Could you check a few things on this model? Use its own coordinates, in mm. Face numbers are marked on the shaded views. A direction names the side the tool comes from. Coordinates: 2 decimals unless noted, no trailing zeros. Write each loop counter-clockwise with the first axis right and the second up, starting at its lowest first coordinate (ties: lowest second). Pieces come first, ordered by that corner, then holes.
Item 1: I want a section at C-C on x = 10.9. Please give me the cut outline in (y, z).
Item 2: Which directions (+Z, -Z, +X, -X, +Y, -Y) give clear straight access to the entire face, cutting with the end or side of a thin tool? Please do the marked faces 5, 6 and 7.
Item 3: For P1, Ø3, axis at y = -27, z = 10.5, coming from the +X side; P2, Ø1.2, axis at y = -17, z = 11.5, coming from the +X side; P3, Ø1.2, axis at y = -16.5, z = 10, coming from the -X side, each with a flat end and sliding along its axis, tell me the tip position at first contact or that it passes through.
Item 4: I want a section at B-B on y = -21.5. Please give me the cut outline in (x, z), then the cut area to 3 significant figures.
Item 5: I want a section at D-D on x = 3.5. Please give me the cut outline in (y, z).
Item 6: I want a section at A-A on x = 19.5. Please give me the cut outline in (y, z).
Item 7: Thinking about a two-plate mould opening in Z: for the marked faces 1, 2, 3 and 4, which applies, +Z half, -Z half, draft (parallel to the pull), parting line (faces both ways), or undercut?
Item 8: If I drill on probe 1 along X at (y, z) = (-10, 10.9); probe 2 along Y at (x, z) = (7.2, 10.9); probe 3 along X at (y, z) = (-11, 14.5), over which ranges is the centre line in solid material (lowest first)?
from build123d import *

# Parameters (mm, degrees)
CROQUIS1_W              = 21.8
CROQUIS1_H              = 35
SALIENTE_EXTRUIR1_DEPTH = 21.8
CROQUIS6_R              = 2
CORTAR_EXTRUIR2_DEPTH   = 21.8
REDONDEO2_R             = 1
REDONDEO3_R             = 4
CROQUIS7_R              = 3.5
CORTAR_EXTRUIR3_DEPTH   = 3
CORTAR_EXTRUIR4_REACH   = 48.642
CROQUIS11_R             = 3.5
CROQUIS11_W             = 3
CROQUIS11_H             = 8.4
MATRIZL1_COUNT          = 2
MATRIZL1_PITCH          = 18.8
CROQUIS14_W             = 3
CROQUIS14_H             = 8.4
SALIENTE_EXTRUIR2_DEPTH = 20
CROQUIS15_W             = 3
CROQUIS15_H             = 8.4
SALIENTE_EXTRUIR3_DEPTH = 20


with BuildPart() as part:
    # Croquis1 → Saliente-Extruir1 (new body)
    with BuildSketch(Plane(origin=(0, 0, 0), x_dir=(0, 0, -1), z_dir=(1, 0, 0))):
        with Locations((-10.9, -17.5)):
            Rectangle(CROQUIS1_W, CROQUIS1_H)
    extrude(amount=SALIENTE_EXTRUIR1_DEPTH)

    # Croquis6 → Cortar-Extruir2 (cut)
    with BuildSketch(Plane.ZY):
        with Locations((10.9, -28)):
            Circle(CROQUIS6_R)
        with Locations((10.9, -17.5)):
            Circle(CROQUIS6_R)
        with Locations(Location((10.9, -7, 0), (0, 0, 180))):
            Circle(CROQUIS6_R)
    extrude(amount=-CORTAR_EXTRUIR2_DEPTH, mode=Mode.SUBTRACT)

    # Redondeo2
    redondeo2_edges = [part.edges().sort_by_distance(p)[0] for p in [
        (21.8, -35, 10.9),
        (21.8, -17.5, 0),
        (21.8, 0, 10.9),
        (0, -17.5, 0),
        (0, -35, 10.9),
        (0, -17.5, 21.8),
        (0, 0, 10.9),
        (21.8, -17.5, 21.8),
    ]]
    fillet(redondeo2_edges, radius=REDONDEO2_R)

    # Redondeo3
    # the kernel refuses this fillet: 4 mm, written as the material it takes off along each edge
    with BuildSketch(Plane(origin=(0, -4, 4), x_dir=(0, 1, 0), z_dir=(0, 0, 1))) as redondeo3_piece_1:
        with BuildLine():
            CenterArc((3, -1), 1, 0, 90)
            Line((4, -1), (4, 0))
            Line((4, 0), (3, 0))
        make_face()
    revolve(axis=Axis((0, -4, 4), (-1, 0, 0)), revolution_arc=90, mode=Mode.SUBTRACT)
    with BuildSketch(Plane(origin=(0, -31, 4), x_dir=(0, 0, -1), z_dir=(0, 1, 0))) as redondeo3_piece_2:
        with BuildLine():
            CenterArc((3, -1), 1, 0, 90)
            Line((4, -1), (4, 0))
            Line((4, 0), (3, 0))
        make_face()
    revolve(axis=Axis((0, -31, 4), (-1, 0, 0)), revolution_arc=90, mode=Mode.SUBTRACT)
    with BuildSketch(Plane(origin=(0, -4, 17.8), x_dir=(0, 0, 1), z_dir=(0, -1, 0))) as redondeo3_piece_3:
        with BuildLine():
            CenterArc((3, -1), 1, 0, 90)
            Line((4, -1), (4, 0))
            Line((4, 0), (3, 0))
        make_face()
    revolve(axis=Axis((0, -4, 17.8), (-1, 0, 0)), revolution_arc=90, mode=Mode.SUBTRACT)
    with BuildSketch(Plane(origin=(0, -31, 17.8), x_dir=(0, -1, 0), z_dir=(0, 0, -1))) as redondeo3_piece_4:
        with BuildLine():
            CenterArc((3, -1), 1, 0, 90)
            Line((4, -1), (4, 0))
            Line((4, 0), (3, 0))
        make_face()
    revolve(axis=Axis((0, -31, 17.8), (-1, 0, 0)), revolution_arc=90, mode=Mode.SUBTRACT)
    with BuildSketch(Plane(origin=(21.8, -4, 4), x_dir=(0, 0, -1), z_dir=(0, -1, 0))) as redondeo3_piece_5:
        with BuildLine():
            CenterArc((3, -1), 1, 0, 90)
            Line((4, -1), (4, 0))
            Line((4, 0), (3, 0))
        make_face()
    revolve(axis=Axis((21.8, -4, 4), (1, 0, 0)), revolution_arc=90, mode=Mode.SUBTRACT)
    with BuildSketch(Plane(origin=(21.8, -31, 4), x_dir=(0, -1, 0), z_dir=(0, 0, 1))) as redondeo3_piece_6:
        with BuildLine():
            CenterArc((3, -1), 1, 0, 90)
            Line((4, -1), (4, 0))
            Line((4, 0), (3, 0))
        make_face()
    revolve(axis=Axis((21.8, -31, 4), (1, 0, 0)), revolution_arc=90, mode=Mode.SUBTRACT)
    with BuildSketch(Plane(origin=(21.8, -4, 17.8), x_dir=(0, 1, 0), z_dir=(0, 0, -1))) as redondeo3_piece_7:
        with BuildLine():
            CenterArc((3, -1), 1, 0, 90)
            Line((4, -1), (4, 0))
            Line((4, 0), (3, 0))
        make_face()
    revolve(axis=Axis((21.8, -4, 17.8), (1, 0, 0)), revolution_arc=90, mode=Mode.SUBTRACT)
    with BuildSketch(Plane(origin=(21.8, -31, 17.8), x_dir=(0, 0, 1), z_dir=(0, 1, 0))) as redondeo3_piece_8:
        with BuildLine():
            CenterArc((3, -1), 1, 0, 90)
            Line((4, -1), (4, 0))
            Line((4, 0), (3, 0))
        make_face()
    revolve(axis=Axis((21.8, -31, 17.8), (1, 0, 0)), revolution_arc=90, mode=Mode.SUBTRACT)
    with BuildSketch(Plane(origin=(0, -35, 21.8), x_dir=(0, 1, 0), z_dir=(1, 0, 0)), Plane(origin=(0, 0, 21.8), x_dir=(0, 0, -1), z_dir=(1, 0, 0))) as redondeo3_piece_9:
        with BuildLine():
            CenterArc((REDONDEO3_R, -REDONDEO3_R), REDONDEO3_R, 90, 90)
            Line((0, -REDONDEO3_R), (0, 0))
            Line((0, 0), (REDONDEO3_R, 0))
        make_face()
    extrude(amount=21.8, mode=Mode.SUBTRACT)
    with BuildSketch(Plane(origin=(0, 0, 0), x_dir=(0, 0, 1), z_dir=(1, 0, 0)), Plane(origin=(0, -35, 0), x_dir=(0, 1, 0), z_dir=(1, 0, 0))) as redondeo3_piece_10:
        with BuildLine():
            CenterArc((REDONDEO3_R, REDONDEO3_R), REDONDEO3_R, 180, 90)
            Line((0, REDONDEO3_R), (0, 0))
            Line((0, 0), (REDONDEO3_R, 0))
        make_face()
    extrude(amount=21.8, mode=Mode.SUBTRACT)

    # Croquis7 → Cortar-Extruir3 (cut)
    with BuildSketch(Plane(origin=(21.8, 0, 0), x_dir=(0, 0, -1), z_dir=(1, 0, 0))):
        with Locations((-10.9, -28)):
            Circle(CROQUIS7_R)
        with Locations((-10.9, -17.5)):
            Circle(CROQUIS7_R)
        with Locations(Location((-10.9, -7, 0), (0, 0, 180))):
            Circle(CROQUIS7_R)
    cortar_extruir3 = extrude(amount=-CORTAR_EXTRUIR3_DEPTH, mode=Mode.SUBTRACT)

    # Croquis11 → Cortar-Extruir4 (cut, up to next)
    with BuildSketch(Plane.XZ.offset(35), mode=Mode.PRIVATE) as cortar_extruir4_sk1:
        with Locations(Location((10.9, 10.9, 0), (0, 0, 270))):
            Circle(CROQUIS11_R)
    cortar_extruir4_tool1 = extrude(cortar_extruir4_sk1.sketch, amount=-CORTAR_EXTRUIR4_REACH, mode=Mode.PRIVATE) & part.part
    # Croquis11 → Cortar-Extruir4 (cut, up to next)
    with BuildSketch(Plane.XZ.offset(35), mode=Mode.PRIVATE) as cortar_extruir4_sk2:
        with Locations((5.4, 10.9)):
            Rectangle(CROQUIS11_W, CROQUIS11_H)
    cortar_extruir4_tool2 = extrude(cortar_extruir4_sk2.sketch, amount=-CORTAR_EXTRUIR4_REACH, mode=Mode.PRIVATE) & part.part
    # Croquis11 → Cortar-Extruir4 (cut, up to next)
    with BuildSketch(Plane.XZ.offset(35), mode=Mode.PRIVATE) as cortar_extruir4_sk3:
        with Locations((16.4, 10.9)):
            Rectangle(CROQUIS11_W, CROQUIS11_H)
    cortar_extruir4_tool3 = extrude(cortar_extruir4_sk3.sketch, amount=-CORTAR_EXTRUIR4_REACH, mode=Mode.PRIVATE) & part.part
    add(cortar_extruir4_tool1.solids().sort_by_distance((10.9, -35, 10.9))[0], mode=Mode.SUBTRACT)
    add(cortar_extruir4_tool2.solids().sort_by_distance((5.4, -35, 10.9))[0], mode=Mode.SUBTRACT)
    add(cortar_extruir4_tool3.solids().sort_by_distance((16.4, -35, 10.9))[0], mode=Mode.SUBTRACT)

    # MatrizL1: Cortar-Extruir3 ×2
    with Locations(*[(-i * MATRIZL1_PITCH, 0, 0) for i in range(1, MATRIZL1_COUNT)]):
        add(cortar_extruir3, mode=Mode.SUBTRACT)

    # Croquis14 → Saliente-Extruir2 (add)
    with BuildSketch(Plane(origin=(0, 0, 0), x_dir=(1, 0, 0), z_dir=(0, 1, 0))):
        with Locations((16.4, -10.9)):
            Rectangle(CROQUIS14_W, CROQUIS14_H)
    extrude(amount=-SALIENTE_EXTRUIR2_DEPTH)

    # Croquis15 → Saliente-Extruir3 (add)
    with BuildSketch(Plane.XZ.offset(35)):
        with Locations((5.4, 10.9)):
            Rectangle(CROQUIS15_W, CROQUIS15_H)
    extrude(amount=-SALIENTE_EXTRUIR3_DEPTH)


solid = part.part
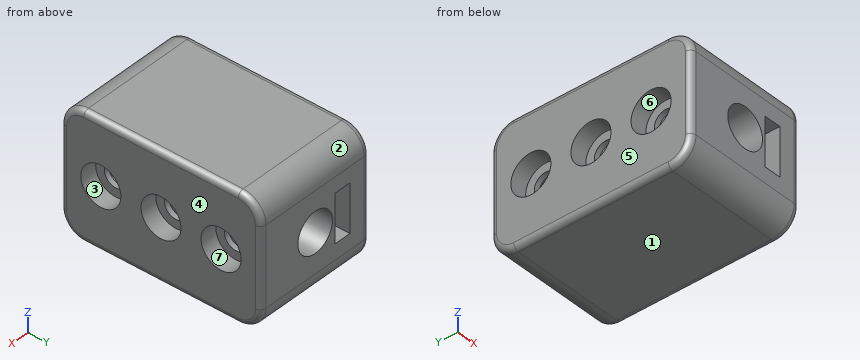
Response values:
1. outline: (-35, 4) arc R4 ccw to (-31, 0) - (-4, 0) arc R4 ccw to (0, 4) - (0, 7.4) - (-35, 7.4) - close; (-35, 14.4) - (0, 14.4) - (0, 17.8) arc R4 ccw to (-4, 21.8) - (-31, 21.8) arc R4 ccw to (-35, 17.8) - close
2. face 5: +Z, -Z, -X, +Y, -Y
2. face 6: -X
2. face 7: +X
3. P1: stops at x = 18.8
3. P2: stops at x = 17.9
3. P3: stops at x = 3.9
4. outline: (0, 1) arc R1 ccw to (1, 0) - (20.8, 0) arc R1 ccw to (21.8, 1) - (21.8, 20.8) arc R1 ccw to (20.8, 21.8) - (1, 21.8) arc R1 ccw to (0, 20.8) - close; hole circle Ø7 at (10.9, 10.9); hole (14.9, 6.7) - (17.9, 6.7) - (17.9, 15.1) - (14.9, 15.1) - close
4. area: 411 mm2
5. outline: (-35, 4) arc R4 ccw to (-31, 0) - (-4, 0) arc R4 ccw to (0, 4) - (0, 17.8) arc R4 ccw to (-4, 21.8) - (-31, 21.8) arc R4 ccw to (-35, 17.8) - close; hole circle Ø4 at (-28, 10.9); hole circle Ø4 at (-17.5, 10.9); hole circle Ø4 at (-7, 10.9)
6. outline: (-35, 4) arc R4 ccw to (-31, 0) - (-4, 0) arc R4 ccw to (0, 4) - (0, 17.8) arc R4 ccw to (-4, 21.8) - (-31, 21.8) arc R4 ccw to (-35, 17.8) - close; hole circle Ø7 at (-28, 10.9); hole circle Ø7 at (-17.5, 10.9); hole circle Ø7 at (-7, 10.9)
7. face 1: -Z half
7. face 2: +Z half
7. face 3: undercut
7. face 4: draft
8. probe 1: x = 3 to 3.9, 6.9 to 7.4, 14.4 to 18.8
8. probe 2: y = -35 to -30, -26 to -19.5, -15.5 to -9, -5 to 0
8. probe 3: x = 0 to 3.9, 6.9 to 21.8
